Autodesk Inventor part; units mm, degrees
ref_plane "YZ Plane" through (0, 0, 0) normal (1, 0, 0) x (0, 1, 0)
ref_plane "XZ Plane" through (0, 0, 0) normal (0, 1, 0) x (-1, 0, 0)
ref_plane "XY Plane" through (0, 0, 0) normal (0, 0, 1) x (1, 0, 0)
sketch "CONTOURS" plane through (0, 0, 0) normal (0, 0, 1) x (1, 0, 0)
  arc A0 (1666.9081, 1038.1557) -> (1691.4363, 1042.062) centre (1677.7135, 1049.2684) ccw
  line L0 (1691.4363, 1042.062) -> (1699.2902, 1057.0177)
  arc A1 (1721.6776, 1061.1873) -> (1699.2902, 1057.0177) centre (1712.1278, 1050.2762) ccw
  line L1 (1721.6776, 1061.1873) -> (1841.3986, 956.4017)
  arc A2 (1839.5956, 933.2336) -> (1841.3986, 956.4017) centre (1831.8487, 945.4907) ccw
  line L2 (1839.5956, 933.2336) -> (1816.9578, 918.9257)
  line L3 (1814.4335, 894.7106) -> (1850.0806, 860.0494)
  arc A3 (22.5497, 860.0494) -> (1850.0806, 860.0494) centre (936.3152, 1749.5593) ccw
  line L4 (22.5497, 860.0494) -> (270.4859, 1042.1379)
  arc A4 (270.4859, 1042.1379) -> (1632.304, 1071.8026) centre (936.3091, 1749.5157) ccw
  line L5 (1632.304, 1071.8026) -> (1666.9081, 1038.1557)
  arc A5 (1816.9578, 918.9257) -> (1814.4335, 894.7106) centre (1825.2389, 905.8233) ccw
  dimension "d1" = 1275.2235
  dimension "d3" = 971.4442
sketch "HOLES" plane through (0, 0, 0) normal (0, 0, 1) x (1, 0, 0)
  line L0 (1808.3556, 951.863) -> (1800.895, 943.7797)
  arc A0 (1795.2427, 943.5532) -> (1800.895, 943.7797) centre (1797.9556, 946.4926) ccw
  line L1 (1795.2427, 943.5532) -> (1715.1445, 1017.4807)
  arc A1 (1714.9181, 1023.1331) -> (1715.1445, 1017.4807) centre (1717.8574, 1020.4201) ccw
  line L2 (1714.9181, 1023.1331) -> (1722.3786, 1031.2164)
  arc A2 (1728.031, 1031.4428) -> (1722.3786, 1031.2164) centre (1725.318, 1028.5034) ccw
  line L3 (1728.031, 1031.4428) -> (1808.1291, 957.5153)
  arc A3 (1808.3556, 951.863) -> (1808.1291, 957.5153) centre (1805.4162, 954.5759) ccw
  line L4 (543.0858, 821.5545) -> (547.6833, 831.5476)
  arc A4 (547.6833, 831.5476) -> (545.7213, 836.8533) centre (544.0494, 833.2195) ccw
  line L5 (545.7213, 836.8533) -> (513.0165, 851.8999)
  arc A5 (513.0165, 851.8999) -> (507.7108, 849.9379) centre (511.3447, 848.266) ccw
  line L6 (507.7108, 849.9379) -> (503.1133, 839.9447)
  arc A6 (503.1133, 839.9447) -> (505.0753, 834.639) centre (506.7471, 838.2729) ccw
  line L7 (505.0753, 834.639) -> (537.7801, 819.5925)
  arc A7 (537.7801, 819.5925) -> (543.0858, 821.5545) centre (539.4519, 823.2264) ccw
  line L8 (481.0423, 782.4016) -> (435.4847, 683.3788)
  arc A8 (435.4847, 683.3788) -> (437.4468, 678.0731) centre (439.1186, 681.7069) ccw
  line L9 (437.4468, 678.0731) -> (447.4399, 673.4755)
  arc A9 (447.4399, 673.4755) -> (452.7456, 675.4376) centre (449.1117, 677.1094) ccw
  line L10 (452.7456, 675.4376) -> (498.3031, 774.4603)
  arc A10 (498.3031, 774.4603) -> (496.3411, 779.766) centre (494.6693, 776.1322) ccw
  line L11 (496.3411, 779.766) -> (486.348, 784.3636)
  arc A11 (486.348, 784.3636) -> (481.0423, 782.4016) centre (484.6762, 780.7297) ccw
  line L12 (446.1185, 610.7891) -> (441.521, 600.7959)
  arc A12 (436.2153, 598.8339) -> (441.521, 600.7959) centre (437.8871, 602.4678) ccw
  line L13 (436.2153, 598.8339) -> (403.5105, 613.8804)
  arc A13 (401.5485, 619.1861) -> (403.5105, 613.8804) centre (405.1824, 617.5143) ccw
  line L14 (401.5485, 619.1861) -> (406.1461, 629.1793)
  arc A14 (411.4518, 631.1413) -> (406.1461, 629.1793) centre (409.7799, 627.5074) ccw
  line L15 (411.4518, 631.1413) -> (444.1565, 616.0948)
  arc A15 (446.1185, 610.7891) -> (444.1565, 616.0948) centre (442.4847, 612.4609) ccw
sketch "LETTERS" plane through (0, 0, 0) normal (0, 0, 1) x (1, 0, 0)
  line L0 (578.69, 694.1928) -> (578.8133, 694.0526)
  line L1 (578.8133, 694.0526) -> (578.9339, 693.9068)
  line L2 (578.9339, 693.9068) -> (579.0516, 693.7555)
  line L3 (579.0516, 693.7555) -> (579.1661, 693.5988)
  line L4 (579.1661, 693.5988) -> (579.2775, 693.4368)
  line L5 (579.2775, 693.4368) -> (579.3854, 693.2696)
  line L6 (579.3854, 693.2696) -> (579.4899, 693.0974)
  line L7 (579.4899, 693.0974) -> (579.5907, 692.9201)
  line L8 (579.5907, 692.9201) -> (579.6877, 692.7381)
  line L9 (579.6877, 692.7381) -> (579.7809, 692.5514)
  line L10 (579.7809, 692.5514) -> (579.87, 692.3601)
  line L11 (579.87, 692.3601) -> (579.955, 692.1646)
  line L12 (579.955, 692.1646) -> (580.0358, 691.9649)
  line L13 (580.0358, 691.9649) -> (580.1123, 691.7612)
  line L14 (580.1123, 691.7612) -> (580.1844, 691.5538)
  line L15 (580.1844, 691.5538) -> (580.252, 691.3428)
  line L16 (580.252, 691.3428) -> (580.3151, 691.1284)
  line L17 (580.3151, 691.1284) -> (580.3736, 690.911)
  line L18 (580.3736, 690.911) -> (580.4275, 690.6906)
  line L19 (580.4275, 690.6906) -> (580.4767, 690.4676)
  line L20 (580.4767, 690.4676) -> (580.5212, 690.2422)
  line L21 (580.5212, 690.2422) -> (580.561, 690.0145)
  line L22 (580.561, 690.0145) -> (580.596, 689.7849)
  line L23 (580.596, 689.7849) -> (580.6263, 689.5536)
  line L24 (580.6263, 689.5536) -> (580.6519, 689.3209)
  line L25 (580.6519, 689.3209) -> (580.6728, 689.0869)
  line L26 (580.6728, 689.0869) -> (580.689, 688.8519)
  line L27 (580.689, 688.8519) -> (580.7006, 688.6162)
  line L28 (580.7006, 688.6162) -> (580.7076, 688.3799)
  line L29 (580.7076, 688.3799) -> (580.71, 688.1435)
  line L30 (580.71, 688.1435) -> (580.7083, 687.9072)
  line L31 (580.7083, 687.9072) -> (580.7019, 687.6709)
  line L32 (580.7019, 687.6709) -> (580.6911, 687.4349)
  line L33 (580.6911, 687.4349) -> (580.6761, 687.1997)
  line L34 (580.6761, 687.1997) -> (580.6569, 686.9652)
  line L35 (580.6569, 686.9652) -> (580.6064, 686.4997)
  line L36 (580.6064, 686.4997) -> (580.5405, 686.0398)
  line L37 (580.5405, 686.0398) -> (580.46, 685.5872)
  line L38 (580.46, 685.5872) -> (580.3659, 685.1429)
  line L39 (580.3659, 685.1429) -> (580.259, 684.7083)
  line L40 (580.259, 684.7083) -> (580.1405, 684.2843)
  line L41 (580.1405, 684.2843) -> (580.0089, 683.8641)
  line L42 (580.0089, 683.8641) -> (579.8616, 683.4415)
  line L43 (579.8616, 683.4415) -> (579.6986, 683.0176)
  line L44 (579.6986, 683.0176) -> (579.5194, 682.5942)
  line L45 (579.5194, 682.5942) -> (579.3242, 682.1727)
  line L46 (579.3242, 682.1727) -> (579.1129, 681.7548)
  line L47 (579.1129, 681.7548) -> (579.0013, 681.5478)
  line L48 (579.0013, 681.5478) -> (578.8857, 681.3423)
  line L49 (578.8857, 681.3423) -> (578.7662, 681.1386)
  line L50 (578.7662, 681.1386) -> (578.6428, 680.9369)
  line L51 (578.6428, 680.9369) -> (578.5156, 680.7375)
  line L52 (578.5156, 680.7375) -> (578.3847, 680.5405)
  line L53 (578.3847, 680.5405) -> (578.2502, 680.3462)
  line L54 (578.2502, 680.3462) -> (578.1121, 680.1549)
  line L55 (578.1121, 680.1549) -> (577.9704, 679.9667)
  line L56 (577.9704, 679.9667) -> (577.8254, 679.7818)
  line L57 (577.8254, 679.7818) -> (577.6772, 679.6006)
  line L58 (577.6772, 679.6006) -> (577.5257, 679.4231)
  line L59 (577.5257, 679.4231) -> (577.3713, 679.2497)
  line L60 (577.3713, 679.2497) -> (577.2139, 679.0805)
  line L61 (577.2139, 679.0805) -> (577.0538, 678.9157)
  line L62 (577.0538, 678.9157) -> (576.891, 678.7555)
  line L63 (576.891, 678.7555) -> (576.7258, 678.6)
  line L64 (576.7258, 678.6) -> (576.5582, 678.4496)
  line L65 (576.5582, 678.4496) -> (576.3886, 678.3042)
  line L66 (576.3886, 678.3042) -> (576.2169, 678.1641)
  line L67 (576.2169, 678.1641) -> (576.0434, 678.0295)
  line L68 (576.0434, 678.0295) -> (575.8683, 677.9003)
  line L69 (575.8683, 677.9003) -> (575.6918, 677.7769)
  line L70 (575.6918, 677.7769) -> (575.5139, 677.6592)
  line L71 (575.5139, 677.6592) -> (575.335, 677.5474)
  line L72 (575.335, 677.5474) -> (575.1552, 677.4416)
  line L73 (575.1552, 677.4416) -> (574.9746, 677.3418)
  line L74 (574.9746, 677.3418) -> (574.7935, 677.2481)
  line L75 (574.7935, 677.2481) -> (574.612, 677.1606)
  line L76 (574.612, 677.1606) -> (574.4304, 677.0792)
  line L77 (574.4304, 677.0792) -> (574.2488, 677.004)
  line L78 (574.2488, 677.004) -> (574.0674, 676.9351)
  line L79 (574.0674, 676.9351) -> (573.8863, 676.8723)
  line L80 (573.8863, 676.8723) -> (573.7057, 676.8158)
  line L81 (573.7057, 676.8158) -> (573.5259, 676.7654)
  line L82 (573.5259, 676.7654) -> (573.3469, 676.7211)
  line L83 (573.3469, 676.7211) -> (573.1689, 676.6829)
  line L84 (573.1689, 676.6829) -> (572.9922, 676.6507)
  line L85 (572.9922, 676.6507) -> (572.8167, 676.6245)
  line L86 (572.8167, 676.6245) -> (572.6427, 676.6042)
  line L87 (572.6427, 676.6042) -> (572.4703, 676.5896)
  line L88 (572.4703, 676.5896) -> (572.2997, 676.5808)
  line L89 (572.2997, 676.5808) -> (572.1309, 676.5775)
  line L90 (572.1309, 676.5775) -> (571.964, 676.5797)
  line L91 (571.964, 676.5797) -> (571.7993, 676.5872)
  line L92 (571.7993, 676.5872) -> (571.6367, 676.6)
  line L93 (571.6367, 676.6) -> (571.4764, 676.6179)
  line L94 (571.4764, 676.6179) -> (571.3185, 676.6407)
  line L95 (571.3185, 676.6407) -> (571.163, 676.6683)
  line L96 (571.163, 676.6683) -> (571.0101, 676.7007)
  line L97 (571.0101, 676.7007) -> (570.8598, 676.7375)
  line L98 (570.8598, 676.7375) -> (570.7121, 676.7787)
  line L99 (578.4356, 694.4565) -> (578.564, 694.3275)
  line L100 (578.3049, 694.5797) -> (578.4356, 694.4565)
  line L101 (578.172, 694.6973) -> (578.3049, 694.5797)
  line L102 (578.0372, 694.8092) -> (578.172, 694.6973)
  line L103 (577.9006, 694.9153) -> (578.0372, 694.8092)
  line L104 (577.7623, 695.0157) -> (577.9006, 694.9153)
  line L105 (577.6225, 695.1104) -> (577.7623, 695.0157)
  line L106 (577.4814, 695.1995) -> (577.6225, 695.1104)
  line L107 (577.3392, 695.2829) -> (577.4814, 695.1995)
  line L108 (577.1959, 695.3608) -> (577.3392, 695.2829)
  line L109 (577.0518, 695.4331) -> (577.1959, 695.3608)
  line L110 (576.9069, 695.5) -> (577.0518, 695.4331)
  line L111 (576.7615, 695.5616) -> (576.9069, 695.5)
  line L112 (576.6156, 695.6178) -> (576.7615, 695.5616)
  line L113 (576.4695, 695.6688) -> (576.6156, 695.6178)
  line L114 (576.3232, 695.7147) -> (576.4695, 695.6688)
  line L115 (569.8928, 698.0178) -> (576.3232, 695.7147)
  line L116 (563.2082, 679.3542) -> (569.8928, 698.0178)
  line L117 (570.7121, 676.7787) -> (563.2082, 679.3542)
  line L118 (578.564, 694.3275) -> (578.69, 694.1928)
extrude "Extrusion2" add sketch "CONTOURS" along normal blind 18
extrude "Extrusion3" cut sketch "HOLES" along normal blind 18
properties part number "Platform D1" material "Wood (Birch)"
Geometry check sheet. Reference: the model listing, model coordinates, mm. A direction names the side the tool comes from. Give positions to 0.01 mm unless a question says otherwise; leave off trailing zeros. Order: outer loops, then holes, each group sorted by start corner. A loop starts at its lowest first (then second) coordinate and runs counter-clockwise, first axis right, second up.
1. Depth check by flat-ended pin: pin 1 (8 mm diameter, centred on y = 571, z = 16, fed in from -X); pin 2 (2 mm diameter, centred on x = 344.5, z = 11.5, fed in from -Y); pin 3 (10 mm diameter, centred on x = 457, z = 4, fed in from -Y). Enter the tip coordinate at first touch or a pass-through.
Completed:
pin 1: stops at x = 439.72
pin 2: stops at y = 619.46
pin 3: stops at y = 565.83
2. Sectioned sample at B-B (y = 985). Record the boundary of the cut face in (x, z), then the cut area to 3 significant figures.
Completed:
outline: (192.69, 0) - (336.96, 0) - (336.96, 18) - (192.69, 18) - close; (1535.66, 0) - (1750.34, 0) - (1750.34, 18) - (1535.66, 18) - close; (1778.35, 0) - (1808.72, 0) - (1808.72, 18) - (1778.35, 18) - close
area: 7,010 mm2
3. Sectioned sample at C-C (z = 4). State how many separate pieces and enclosed holes the cut face has, then the cut area to 3 significant figures.
Completed:
separate pieces: 1
enclosed holes: 4
area: 543,000 mm2
4. Scan lines: line 1 (X direction, y = 877, z = 12); line 2 (X direction, y = 718.5, z = 12.5); line 3 (Y direction, x = 509, z = 5.25). Record each from-to range of solid material in increasing order.
Completed:
line 1: x = 45.63 to 509.2, 1363.42 to 1832.65
line 2: x = 185.91 to 451.64, 472.56 to 1686.72
line 3: y = 548.06 to 832.83, 851.51 to 877.1
5. Access from +Z, -Z, +X, -X, +Y, -Y to the whole of each face (thin tool, end or side, straight path). Record for faces 1 (the face through (1832.01, 877.62, 8.87)), 2 (the face through (1780.7, 1009.53, 8.87)), 3 (the face through (475.205, 724.256, 8.874)), 4 (the face through (1649.364, 1055.215, 8.874)).
Completed:
face 1: +Z, -Z, +X
face 2: +Z, -Z, +X, +Y
face 3: +Z, -Z
face 4: +Z, -Z, +Y
6. Draft check along Y on faces 5 (the face through (458.58, 733.58, 8.87)), 6 (the face through (924, 777, 0)), 7 (the face through (144.782, 949.819, 8.874)). Enter one of: pulls with the +Y half, pulls with the -Y half, needs draft (parallel to the pull), parting line crosses it, or undercut.
Completed:
face 5: undercut
face 6: needs draft
face 7: pulls with the +Y half
7. Sectioned sample at A-A (y = 753). Record the boundary of the cut face in (x, z), then the cut area to 3 significant figures.
Completed:
outline: (140.66, 0) - (467.52, 0) - (467.52, 18) - (140.66, 18) - close; (488.43, 0) - (1731.97, 0) - (1731.97, 18) - (488.43, 18) - close
area: 28,300 mm2
8. Sectioned sample at D-D (y = 875.5). Record the boundary of the cut face in (x, z).
Completed:
outline: (43.59, 0) - (512.28, 0) - (512.28, 18) - (43.59, 18) - close; (1360.34, 0) - (1834.19, 0) - (1834.19, 18) - (1360.34, 18) - close
